Autodesk Fusion 360 part; units mm, degrees
sketch "Sketch1" plane through (0, 0, 0) normal (0, 0, 1) x (1, 0, 0)
  line L0 (0, 0) -> (82, 0)
  line L1 (82, 0) -> (82, 43)
  line L2 (82, 43) -> (0, 43)
  line L3 (0, 43) -> (0, 0)
  dimension "d1" = 82
  dimension "d2" = 43
extrude "Extrude1" add sketch "Sketch1" along normal blind 37
sketch "Sketch2" plane through (0, 0, 37) normal (0, 0, 1) x (-1, 0, 0)
  line L0 (0, -43) -> (0, 0)
  line L1 (0, 0) -> (-82, 0)
  line L2 (-82, 0) -> (-82, -43)
  line L3 (-82, -43) -> (0, -43)
  line L4 (-3, -3) -> (-79, -3)
  line L5 (-79, -3) -> (-79, -40)
  line L6 (-79, -40) -> (-3, -40)
  line L7 (-3, -40) -> (-3, -3)
  dimension "d5" = 3
  dimension "d6" = 3
  dimension "d7" = 3
  dimension "d8" = 3
extrude "Extrude2" cut sketch "Sketch2" against normal blind 34 contours L4 L5 L6 L7
sketch "Sketch3" plane through (0, 0, 0) normal (-1, 0, 0) x (0, -1, 0)
  line L0 (-43, 0) -> (0, 0)
  line L1 (0, 0) -> (0, 37)
  line L2 (0, 37) -> (-43, 37)
  line L3 (-43, 37) -> (-43, 0)
  circle A0 centre (-21.5, -10) radius 10
  circle A1 centre (-21.5, -10) radius 12.5
  line L4 (-46.7088, -16) -> (3.2912, -16)
  line L5 (-32.4659, -16) -> (-43, 0)
  line L6 (-10.5341, -16) -> (0, 0)
  dimension "d11" = 20
  dimension "d12" = 25
  dimension "d13" = 10
  dimension "d14" = 21.5
  dimension "d16" = 16
extrude "Extrude3" add sketch "Sketch3" against normal blind 82 contours L0 A1 L5 | L0 A0 A1 L4 | L0 A0 A1 L4 | L0 A1 L6
fillet "Fillet1" radius 1.5 6 edges at (41, 13.5, -16) (41, 29.5, -16) (41, 32.4659, -16) (41, 10.5341, -16) (41, 43, 0) (41, 0, 0)
sketch "Sketch4" plane through (0, 0, 0) normal (-1, 0, 0) x (0, -1, 0)
  arc A0 (-0.2472, -0.3754) -> (0, 0.4495) centre (-1.5, 0.4495) ccw
  line L0 (0, 0.4495) -> (0, 37)
  line L1 (0, 37) -> (-43, 37)
  line L2 (-43, 37) -> (-43, 0.4495)
  arc A1 (-43, 0.4495) -> (-42.7528, -0.3754) centre (-41.5, 0.4495) ccw
  line L3 (-42.7528, -0.3754) -> (-33.8235, -13.938)
  arc A2 (-33.8235, -13.938) -> (-31.1266, -12.7071) centre (-32.5706, -13.1131) ccw
  arc A3 (-11.8734, -12.7071) -> (-31.1266, -12.7071) centre (-21.5, -10) ccw
  arc A4 (-11.8734, -12.7071) -> (-9.1765, -13.938) centre (-10.4294, -13.1131) ccw
  line L4 (-9.1765, -13.938) -> (-0.2472, -0.3754)
  line L5 (-29, 34.4495) -> (-3, 34.4495)
  line L6 (-3, 34.4495) -> (-3, 3.4495)
  line L7 (-3, 3.4495) -> (-29, 3.4495)
  line L8 (-29, 3.4495) -> (-29, 34.4495)
  circle A5 centre (-16, 18.9495) radius 12
  circle A6 centre (-25.45, 30.8995) radius 1.75
  circle A7 centre (-6.55, 6.9995) radius 1.75
  line L9 (0, 0.4495) -> (-43, 0.4495)
  line L10 (-31.5, 3.4495) -> (-40, 3.4495)
  line L11 (-40, 3.4495) -> (-40, 19.4495)
  line L12 (-40, 19.4495) -> (-31.5, 19.4495)
  line L13 (-31.5, 19.4495) -> (-31.5, 3.4495)
  dimension "d21" = 24
  dimension "d22" = 31
  dimension "d23" = 26
  dimension "d24" = 13
  dimension "d25" = 15.5
  dimension "d26" = 3.5
  dimension "d27" = 3.5
  dimension "d28" = 3.55
  dimension "d29" = 3.55
  dimension "d30" = 3.55
  dimension "d31" = 3.55
  dimension "d32" = 3
  dimension "d33" = 3
  dimension "d34" = 16
  dimension "d35" = 8.5
  dimension "d36" = 3
  dimension "d37" = 3
extrude "Extrude4" cut sketch "Sketch4" against normal blind 3 contours A5 | A6 | A7 | L10 L11 L12 L13
sketch "Sketch5" plane through (3, 0, 0) normal (1, 0, 0) x (0, 1, 0)
  line L0 (40, 3.4495) -> (31.5, 3.4495)
  line L1 (31.5, 3.4495) -> (31.5, 19.4495)
  line L2 (31.5, 19.4495) -> (40, 19.4495)
  line L3 (40, 19.4495) -> (40, 37)
  line L4 (40, 37) -> (3, 37)
  line L5 (3, 37) -> (3, 3)
  line L6 (3, 3) -> (40, 3)
  line L7 (40, 3) -> (40, 3.4495)
  circle A0 centre (16, 18.9495) radius 12
  circle A1 centre (6.55, 6.9995) radius 1.75
  circle A2 centre (25.45, 30.8995) radius 1.75
  line L8 (40, 3) -> (29.5, 3)
  line L9 (29.5, 3) -> (29.5, 21.4495)
  line L10 (29.5, 21.4495) -> (40, 21.4495)
  line L11 (40, 21.4495) -> (40, 3)
  dimension "d40" = 2
  dimension "d41" = 2
extrude "Extrude5" add sketch "Sketch5" along normal blind 10 contours L0 L1 L2 L3 L6 L7 L8 L9 L10 L11
fillet "Fillet2" radius 1 2 edges at (6.5, 31.5, 19.4495) (6.5, 40, 19.4495)
sketch "Sketch6" plane through (82, 0, 0) normal (1, 0, 0) x (0, 1, 0)
  arc A0 (0, 0.4495) -> (0.2472, -0.3754) centre (1.5, 0.4495) ccw
  line L0 (0.2472, -0.3754) -> (9.1765, -13.938)
  arc A1 (9.1765, -13.938) -> (11.8734, -12.7071) centre (10.4294, -13.1131) ccw
  arc A2 (31.1266, -12.7071) -> (11.8734, -12.7071) centre (21.5, -10) ccw
  arc A3 (31.1266, -12.7071) -> (33.8235, -13.938) centre (32.5706, -13.1131) ccw
  line L1 (33.8235, -13.938) -> (42.7528, -0.3754)
  arc A4 (42.7528, -0.3754) -> (43, 0.4495) centre (41.5, 0.4495) ccw
  line L2 (43, 0.4495) -> (43, 37)
  line L3 (43, 37) -> (0, 37)
  line L4 (0, 37) -> (0, 0.4495)
  circle A5 centre (21.5, 18.725) radius 6
  dimension "d46" = 21.5
  dimension "d47" = 36.5505
  dimension "d48" = 18.275
  dimension "d49" = 12
extrude "Extrude6" cut sketch "Sketch6" against normal blind 3 contours A5
sketch "Sketch7" plane through (0, 0, 37) normal (0, 0, 1) x (-1, 0, 0)
  line L0 (-79, -3) -> (-3, -3)
  line L1 (-3, -3) -> (-3, -40)
  line L2 (-3, -40) -> (-79, -40)
  line L3 (-79, -40) -> (-79, -3)
  line L4 (0, -43) -> (0, 0)
  line L5 (0, 0) -> (-82, 0)
  line L6 (-82, 0) -> (-82, -43)
  line L7 (-82, -43) -> (0, -43)
  circle A0 centre (-2, -2) radius 1
  circle A1 centre (-80, -41) radius 1
  dimension "d52" = 2
  dimension "d53" = 2
  dimension "d54" = 2
  dimension "d55" = 2
  dimension "d56" = 2
  dimension "d57" = 2
extrude "Extrude7" cut sketch "Sketch7" against normal blind 5 contours A0 | A1
equation "d14 = ( 43 / 2 ) * 1 mm"
equation "d24 = ( 26 / 2 ) * 1 mm"
equation "d25 = ( 31 / 2 ) * 1 mm"
equation "d46 = ( 43 / 2 ) * 1 mm"
equation "d48 = ( 36.55 / 2 ) * 1 mm"
Could you check a few things on this model? Use its own coordinates, in mm. A direction names the side the tool comes from. Give positions to 0.01 mm unless a question says otherwise; leave off trailing zeros. Write each loop counter-clockwise with the first axis right and the second up, starting at its lowest first coordinate (ties: lowest second). Pieces come first, ordered by that corner, then holes. Notation, with made-up numbers: (37.25, -34) -> (58.25, -34) arc R13 ccw to (58.25, -17) -> close; hole circle Ø5 at (3.5, 10). An arc over 180 degrees is marked (long way). Write each question's results on one line, items separated by ' | '. Start each with the question number.
Q1. I'm going to push flat-ended pins straight in: pin 1 Ø6 at (x, z) = (44.5, 5.5) entering from -Y; pin 2 Ø10 at (y, z) = (19, 14.5) entering from -X; pin 3 Ø1 at (x, y) = (25.5, 26.5) entering from +Z; pin 4 Ø7 at (x, y) = (9, 34.5) entering from +Z. Where does each tip first touch, or does it pass through?
Q2. Suppose I cut it at B-B, the plane z = -11. List the corners of the cut face in (x, y) for me.
Q3. Suppose I cut it at C-C, the plane y = 41. List the corners of the cut face in (x, z) for me.
Q4. We'd pull the mould along X, two halves only. Please class faces 4 (the face through (1.48, 9.55, 29.07)), 5 (the face through (2, 2, 32)), 6 (the face through (8, 29.5, 12)), 7 (the face through (0, 27, 11)): +X half, -X half, draft (parallel to the pull), parting line (faces both ways), or undercut.
Q5. I need wall thicknesses on probe 1 along Y at (x, z) = (49, 21); probe 2 along Z at (x, y) = (2.35, 25.45); probe 3 along X at (y, z) = (41, 35.8). Which ranges of each line are inside material? Lowest first, please.
Q6. Which directions (+Z, -Z, +X, -X, +Y, -Y) give clear straight access to the entire face, cutting with the end or side of a thin tool? Please do faces 1 (the face through (79, 17, 24)), 2 (the face through (40.426, 38.225, -7.252)), 3 (the face through (6, 36, 19.45)).
Q7. Suppose I cut it at D-D, the plane x = 2. State how many separate pieces and enclosed holes the cut face has, and give its area (3 significant figures).
Q8. Suppose I cut it at A-A, the plane y = 25.45. List the corners of the cut face in (x, z) for me, and give its area (3 significant figures).
Outcome:
1) pin 1: y = 0 | pin 2: x = 79 | pin 3: z = 3 | pin 4: z = 21.45
2) outline: (0, 7.24) -> (82, 7.24) -> (82, 11.55) -> (0, 11.55) -> close; (0, 31.45) -> (82, 31.45) -> (82, 35.76) -> (0, 35.76) -> close
3) outline: (0, -3.04) -> (82, -3.04) -> (82, 37) -> (81, 37) -> (81, 32) -> (79, 32) -> (79, 37) -> (0, 37) -> close
4) face 4: draft | face 5: undercut | face 6: undercut | face 7: -X half
5) probe 1: 0 to 3, 40 to 43 | probe 2: -0.81 to 11.55, 26.35 to 29.15, 32.65 to 37 | probe 3: 0 to 79, 81 to 82
6) face 1: +Z | face 2: -Z, +X, -X, +Y | face 3: -X
7) separate pieces: 1 | enclosed holes: 4 | area: 1,210 mm2
8) outline: (0, -0.81) -> (82, -0.81) -> (82, 14.21) -> (79, 14.21) -> (79, 3) -> (3, 3) -> (3, 11.55) -> (0, 11.55) -> close; (0, 26.35) -> (3, 26.35) -> (3, 29.15) -> (0, 29.15) -> close; (0, 32.65) -> (3, 32.65) -> (3, 37) -> (0, 37) -> close; (79, 23.24) -> (82, 23.24) -> (82, 37) -> (79, 37) -> close | area: 435 mm2
